The model under review builds one solid part; all positions refer to its coordinate system, in mm. Face numbers are marked on the shaded views. A direction names the side the tool comes from. Give positions to 0.01 mm unless a question says otherwise; leave off trailing zeros. Order: outer loops, then holes, each group sorted by start corner. A loop starts at its lowest first (then second) coordinate and runs counter-clockwise, first axis right, second up.
```python
from build123d import *

# Parameters (mm, degrees)
SKETCH1_R           = 16.891
EXTRUDE1_DEPTH      = 7.6
SKETCH2_R           = 9.998276061
EXTRUDE2_DEPTH      = 5.5
SKETCH3_R           = 16.891
EXTRUDE3_DEPTH      = 53.975
SKETCH4_R           = 5.5
BOSS_EXTRUDE1_DEPTH = 15.5
CUT_EXTRUDE1_START  = -9
SKETCH5_R           = 5.5
SKETCH5_R_2         = 5
CUT_EXTRUDE1_DEPTH  = 9
SKETCH6_R           = 7.62
BOSS_EXTRUDE2_DEPTH = 100


with BuildPart() as part:
    # Sketch1 → Extrude1 (new body)
    with BuildSketch(Plane(origin=(0, 0, 0), x_dir=(1, 0, 0), z_dir=(0, 1, 0))):
        with Locations(Location((0, 0, 0), (0, 0, 90))):
            Circle(SKETCH1_R)
    extrude(amount=EXTRUDE1_DEPTH)

    # Sketch2 → Extrude2 (add)
    with BuildSketch(Plane(origin=(0, 7.6, 0), x_dir=(1, 0, 0), z_dir=(0, 1, 0))):
        with Locations(Location((0, 0, 0), (0, 0, 270))):
            Circle(SKETCH2_R)
    extrude(amount=EXTRUDE2_DEPTH)

    # Sketch3 → Extrude3 (add)
    with BuildSketch(Plane(origin=(0, 13.1, 0), x_dir=(1, 0, 0), z_dir=(0, 1, 0))):
        with Locations(Location((0, 0, 0), (0, 0, 90))):
            Circle(SKETCH3_R)
    extrude(amount=EXTRUDE3_DEPTH)

    # Sketch4 → Boss-Extrude1 (add)
    with BuildSketch(Plane.XZ):
        with Locations(Location((0, 0, 0), (0, 0, 90))):
            Circle(SKETCH4_R)
    extrude(amount=BOSS_EXTRUDE1_DEPTH)

    # Sketch5 → Cut-Extrude1 (cut)
    with BuildSketch(Plane.XZ.offset(15.5).offset(CUT_EXTRUDE1_START)):
        with Locations(Location((0, 0, 0), (0, 0, 90))):
            Circle(SKETCH5_R)
        with Locations(Location((0, 0, 0), (0, 0, 270))):
            Circle(SKETCH5_R_2, mode=Mode.SUBTRACT)
    extrude(amount=CUT_EXTRUDE1_DEPTH, mode=Mode.SUBTRACT)

    # Sketch6 → Boss-Extrude2 (add)
    with BuildSketch(Plane(origin=(0, 67.075, 0), x_dir=(-1, 0, 0), z_dir=(0, 1, 0))):
        with Locations(Location((0, 0, 0), (0, 0, 90))):
            Circle(SKETCH6_R)
    extrude(amount=BOSS_EXTRUDE2_DEPTH)


solid = part.part
```
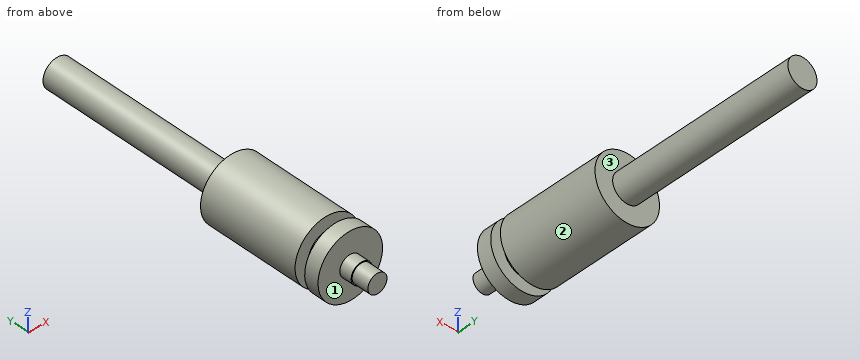
Item 1: Take a section at A-A (x = 0). Give the boundary of the cut face in (y, z) (3 decimals), and give its area (3 significant figures).
Values found:
outline: (-15.5, -5) - (-6.5, -5) - (-6.5, -5.5) - (0, -5.5) - (0, -16.891) - (7.6, -16.891) - (7.6, -9.998) - (13.1, -9.998) - (13.1, -16.891) - (67.075, -16.891) - (67.075, -7.62) - (167.075, -7.62) - (167.075, 7.62) - (67.075, 7.62) - (67.075, 16.891) - (13.1, 16.891) - (13.1, 9.998) - (7.6, 9.998) - (7.6, 16.891) - (0, 16.891) - (0, 5.5) - (-6.5, 5.5) - (-6.5, 5) - (-15.5, 5) - close
area: 3,880 mm2
Item 2: Clearance check with flat-ended pins moving along their axes: pin 1 Ø3 at (y, z) = (104, 2.5) entering from +X; pin 2 Ø8 at (x, y) = (10.5, 6.5) entering from -Z; pin 3 Ø3 at (x, y) = (-11.5, 66) entering from -Z. State where each tip first meets the part, or that it passes through.
Values found:
pin 1: stops at x = 7.55
pin 2: stops at z = -15.59
pin 3: stops at z = -13.61
Item 3: For line 1 (Y direction, x = -3, z = -12) (3 decimals); line 2 (Y direction, x = -1.5, z = 5) (3 decimals); line 3 (Y direction, x = -9.5, z = 2) (3 decimals), list the stretches that pass through material, from the lowest coordinate up.
Values found:
line 1: y = 0 to 7.6, 13.1 to 67.075
line 2: y = -6.5 to 167.075
line 3: y = 0 to 67.075
Item 4: Take a section at D-D (y = 63.5). Give the boundary of the cut face in (x, z).
Values found:
outline: circle Ø33.78 at (0, 0)
Item 5: For the marked faces 1, 2 and 3, list the 3-axis set-ups (+Z, -Z, +X, -X, +Y, -Y) from which the entire face can be reached by the end or side of a thin tool; tool diameter is ignored.
Values found:
face 1: -Y
face 2: +Y, -Y
face 3: +Y
Item 6: Take a section at C-C (x = 13.5). Give the boundary of the cut face in (y, z) (3 decimals), and give its area (3 significant figures).
Values found:
outline: (0, -10.152) - (7.6, -10.152) - (7.6, 10.152) - (0, 10.152) - close; (13.1, -10.152) - (67.075, -10.152) - (67.075, 10.152) - (13.1, 10.152) - close
area: 1,250 mm2
Item 7: Take a section at B-B (z = 0). Give the boundary of the cut face in (x, y) (3 decimals).
Values found:
outline: (-16.891, 0) - (-5.5, 0) - (-5.5, -6.5) - (-5, -6.5) - (-5, -15.5) - (5, -15.5) - (5, -6.5) - (5.5, -6.5) - (5.5, 0) - (16.891, 0) - (16.891, 7.6) - (9.998, 7.6) - (9.998, 13.1) - (16.891, 13.1) - (16.891, 67.075) - (7.62, 67.075) - (7.62, 167.075) - (-7.62, 167.075) - (-7.62, 67.075) - (-16.891, 67.075) - (-16.891, 13.1) - (-9.998, 13.1) - (-9.998, 7.6) - (-16.891, 7.6) - close
